```python
from build123d import *

# Parameters (mm, degrees)
SKETCH1_W           = 100
SKETCH1_H           = 80
BOSS_EXTRUDE1_DEPTH = 50
SKETCH2_R           = 10
SKETCH2_R_2         = 7
BOSS_EXTRUDE2_DEPTH = 20


with BuildPart() as part:
    # Sketch1 → Boss-Extrude1 (new body)
    with BuildSketch(Plane.YZ):
        Rectangle(SKETCH1_W, SKETCH1_H)
    extrude(amount=BOSS_EXTRUDE1_DEPTH)

    # Sketch2 → Boss-Extrude2 (add)
    # profile 1 of 2: a face of its own
    with BuildSketch(Plane.YZ.offset(50)):
        with Locations(Location((-35, 0, 0), (0, 0, 270))):
            Circle(SKETCH2_R)
        with Locations(Location((-35, 0, 0), (0, 0, 270))):
            Circle(SKETCH2_R_2, mode=Mode.SUBTRACT)
    # profile 2 of 2: a face of its own
    with BuildSketch(Plane.YZ.offset(50)):
        with Locations(Location((35, 0, 0), (0, 0, 90))):
            Circle(SKETCH2_R)
        with Locations(Location((35, 0, 0), (0, 0, 90))):
            Circle(SKETCH2_R_2, mode=Mode.SUBTRACT)
    extrude(amount=BOSS_EXTRUDE2_DEPTH)


solid = part.part
```
Build history of the part. All positions in model axes, mm. A direction names the side the tool comes from. Round coordinates to 2 decimals unless told otherwise and drop trailing zeros. Write each loop counter-clockwise with the first axis right and the second up, starting at its lowest first coordinate (ties: lowest second). Pieces come first, ordered by that corner, then holes. Notation, with made-up numbers: (13.5, -2) -> (41.5, -2) arc R21 ccw to (41.5, 16) -> close; hole circle Ø8 at (-38, 52.5). An arc over 180 degrees is marked (long way). Put each result on its own line as item: value.
Item 1: Slice it at A-A, the plane z = 0. Give the cut face in (x, y).
Here are the results:
outline: (0, -50) -> (50, -50) -> (50, -45) -> (70, -45) -> (70, -42) -> (50, -42) -> (50, -28) -> (70, -28) -> (70, -25) -> (50, -25) -> (50, 25) -> (70, 25) -> (70, 28) -> (50, 28) -> (50, 42) -> (70, 42) -> (70, 45) -> (50, 45) -> (50, 50) -> (0, 50) -> close
Item 2: Slice it at D-D, the plane z = -30. Give the cut face in (x, y).
Here are the results:
outline: (0, -50) -> (50, -50) -> (50, 50) -> (0, 50) -> close
Item 3: Flat gauge pins, fed straight in: P1, Ø1, axis at y = 24.5, z = -26.5, coming from the +X side; P2, Ø1.5, axis at x = 52.5, z = 13.5, coming from the +Y side (3 decimals). Where does each tip first touch, or does it go through?
Here are the results:
P1: stops at x = 50
P2: passes through
Item 4: Slice it at C-C, the plane y = 35. Give the cut face in (x, z), plus the area to 3 significant figures.
Here are the results:
outline: (0, -40) -> (50, -40) -> (50, -10) -> (70, -10) -> (70, -7) -> (50, -7) -> (50, 7) -> (70, 7) -> (70, 10) -> (50, 10) -> (50, 40) -> (0, 40) -> close
area: 4,120 mm^2
Item 5: Two-plate mould, pull along Z, no slides. Class faces 1 (the face through (59.86, 44.76, -2.17)), 2 (the face through (25, 50, -1)), 3 (the face through (59.86, 28.06, -0.91)): pulls with the +Z half, pulls with the -Z half, needs draft (parallel to the pull), parting line crosses it, or undercut.
Here are the results:
face 1: parting line crosses it
face 2: needs draft
face 3: undercut
Item 6: Wall check: probe 1 along Y at (x, z) = (56, 0); probe 2 along Z at (x, y) = (62.5, 35); probe 3 along X at (y, z) = (-16.5, -35.5). Give the ranges that are in metal, low to high. Write a range as from..to.
Here are the results:
probe 1: y = -45..-42, -28..-25, 25..28, 42..45
probe 2: z = -10..-7, 7..10
probe 3: x = 0..50
Item 7: Slice it at B-B, the plane x = 61. Give the cut face in (y, z), plus the area to 3 significant figures.
Here are the results:
outline: circle Ø20 at (-35, 0); circle Ø20 at (35, 0); hole circle Ø14 at (-35, 0); hole circle Ø14 at (35, 0)
area: 320 mm^2
Item 8: Tool access for faces 4 (the face through (59.86, -28.06, 0.91)), 5 (the face through (25, -1, 40)): list every direction of +Z, -Z, +X, -X, +Y, -Y with a clear straight run to the whole face (end or side of a thin tool).
Here are the results:
face 4: +X
face 5: +Z, +X, -X, +Y, -Y
